```python
from build123d import *

# Parameters (mm, degrees)
F1_DEPTH = 12.7


# Not quite as in the source:
# - the program builds the solid bodies; features that only make, move or delete a surface that nothing else refers to are left out


with BuildPart() as f1:
    # F0 (on Right) → F1 (new body)
    with BuildSketch(Plane.YZ):
        with BuildLine():
            Line((-22.5137730746, 11.7596777994), (-22.5137730746, 25.4))
            Line((-22.5137730746, 25.4), (-174.9137730746, 25.4))
            Line((-174.9137730746, 25.4), (-174.9137730746, -25.4))
            Line((-174.9137730746, -25.4), (-22.5137730746, -25.4))
            Line((-22.5137730746, -25.4), (-22.5137730746, -11.7596777994))
            ThreePointArc((-22.5137730746, -11.7596777994), (25.4, 0), (-22.5137730746, 11.7596777994))
        make_face()
        Polygon((-12.2498031706, -7.0739961229), (-12.2498031706, 6.2070912682), (0, 6.2070912682), (13.0541240796, 13.2165625691), (13.0541240796, -11.5010300651), (0, -7.0739961229), align=None, mode=Mode.SUBTRACT)
    extrude(amount=F1_DEPTH)


solid = f1.part
```
Source: CAD feature listing. Evaluate the final solid. Frame: model axes, mm. A direction names the side the tool comes from. Give positions to 0.01 mm unless a question says otherwise; leave off trailing zeros. Loops run counter-clockwise (first coordinate to the right, second up) from the corner with the lowest first, then second, coordinate; pieces in that order, holes last. Notation, with made-up numbers: (42.25, -5) - (101.25, -5) arc R26 ccw to (101.25, 15) - close; hole circle Ø2 at (51.25, 54). An arc over 180 degrees is marked (long way). Use CSV: the item, a comma, the result in double quotes. Start each with the question number.
1. Section C-C (z = 17.5). Output: boundary loops of the cut face in (x, y), then the cut area to 3 significant figures.
2. Section A-A (z = 0). Output: boundary loops of the cut face in (x, y), then the cut area to 3 significant figures.
3. Ray query, L1, parallel to Y at x = 2.25, z = 1; L2, parallel to Y at x = 10.5, z = 22.5; L3, parallel to Z at x = 8.5, y = -6. Return the intervals inside material, ascending.
4. Pin query (flat end, axial travel): pin 1 (5 mm diameter, centred on x = 11, z = 14.5, fed in from +Y); pin 2 (4 mm diameter, centred on x = 9.5, z = 18.5, fed in from +Y); pin 3 (5 mm diameter, centred on x = 5.5, y = -9, fed in from -Z). Return the tip coordinate at first contact, or that it passes through.
5. Draft query along Y for faces 1 (the cylindrical face through (6.261, 25.382, -0.946)), 2 (the flat face through (6, -174.914, 0)), 3 (the flat face through (6, -100, -25.4)). Return one class per face: +Y half, -Y half, draft (parallel to the pull), parting line (faces both ways), or undercut.
6. Reachability of faces 4 (the flat face through (0, -98, 0)), 5 (the flat face through (6, -12.25, -1)) from +Z, -Z, +X, -X, +Y, -Y: full face, straight path, thin tool, end or side. Return the list, or none.
7. Section B-B (x = 3.5). Output: boundary loops of the cut face in (y, z).
Response:
1,outline,"(0, -174.91) - (12.7, -174.91) - (12.7, -22.51) - (0, -22.51) - close; (0, -18.41) - (12.7, -18.41) - (12.7, 18.41) - (0, 18.41) - close"
1,area,"2,400 mm²"
2,outline,"(0, -174.91) - (12.7, -174.91) - (12.7, -12.25) - (0, -12.25) - close; (0, 13.05) - (12.7, 13.05) - (12.7, 25.4) - (0, 25.4) - close"
2,area,"2,220 mm²"
3,L1,"-174.91 to -12.25, 13.05 to 25.38"
3,L2,"-174.91 to -22.51, -11.79 to 11.79"
3,L3,"-24.68 to -7.07, 6.21 to 24.68"
4,pin 1,"y = 22.39"
4,pin 2,"y = 19.31"
4,pin 3,"z = -24.55"
5,face 1,"undercut"
5,face 2,"-Y half"
5,face 3,"draft"
6,face 4,"+Z, -Z, -X, +Y, -Y"
6,face 5,"+X, -X"
7,outline,"(-174.91, -25.4) - (-22.51, -25.4) - (-22.51, -11.76) arc R25.4 ccw (long way) to (-22.51, 11.76) - (-22.51, 25.4) - (-174.91, 25.4) - close; hole (-12.25, -7.07) - (0, -7.07) - (13.05, -11.5) - (13.05, 13.22) - (0, 6.21) - (-12.25, 6.21) - close"
